```python
from build123d import *

# Parameters (mm, degrees)
BOSS_EXTRUDE1_DEPTH = 2.5
CUT_EXTRUDE1_REACH  = 26.645
SKETCH2_R           = 1.715
SKETCH2_R_2         = 8.98
SKETCH3_R           = 2.6543
BOSS_EXTRUDE2_DEPTH = 70.305
BOSS_EXTRUDE3_START = 4
SKETCH4_R           = 21
SKETCH4_R_2         = 8.98
BOSS_EXTRUDE3_DEPTH = 4
SKETCH6_R           = 21
SKETCH6_R_2         = 8.98
BOSS_EXTRUDE4_DEPTH = 2
CUT_EXTRUDE3_START  = -15
SKETCH7_R           = 1.715
CUT_EXTRUDE3_DEPTH  = 15
SKETCH8_R           = 8.98
CUT_EXTRUDE4_DEPTH  = 2
SKETCH9_R           = 11.0744
SKETCH9_R_2         = 8.98
BOSS_EXTRUDE5_DEPTH = 2.35


with BuildPart() as part:
    # Sketch1 → Boss-Extrude1 (new body)
    with BuildSketch(Plane(origin=(0, 0, 0), x_dir=(1, 0, 0), z_dir=(0, 1, 0))):
        with BuildLine():
            Line((0.597960958, 12.236443242), (0.597960958, 17.5133))
            Line((0.597960958, 17.5133), (-2.819411684, 17.5133))
            Line((-2.819411684, 17.5133), (-2.819411684, 11.976881697))
            ThreePointArc((-2.819411684, 11.976881697), (-9.752212861, 8.278991937), (-13.533031252, 1.391065316))
            ThreePointArc((-13.533031252, 1.391065316), (-17.156497956, -0.999626805), (-13.683409812, -3.603965207))
            ThreePointArc((-13.683409812, -3.603965207), (-10.042516815, -11.01106651), (-2.819411684, -15.004561697))
            Line((-2.819411684, -15.004561697), (-2.819411684, -17.5133))
            Line((-2.819411684, -17.5133), (0.597960958, -17.5133))
            Line((0.597960958, -17.5133), (0.597960958, -15.264123242))
            ThreePointArc((0.597960958, -15.264123242), (9.161591247, -11.721092084), (13.538839655, -3.55233882))
            ThreePointArc((13.538839655, -3.55233882), (17.156522938, -1.000460972), (13.393344487, 1.331534062))
            ThreePointArc((13.393344487, 1.331534062), (8.853545908, 8.96396608), (0.597960958, 12.236443242))
        make_face()
    extrude(amount=BOSS_EXTRUDE1_DEPTH)

    # Sketch2 → Cut-Extrude1 (cut, up to next)
    with BuildSketch(Plane(origin=(0, 2.5, 0), x_dir=(1, 0, 0), z_dir=(0, 1, 0)), mode=Mode.PRIVATE) as cut_extrude1_sk1:
        with Locations(Location((-14.5034, -1.0795, 0), (0, 0, 270))):
            Circle(SKETCH2_R)
    cut_extrude1_tool1 = extrude(cut_extrude1_sk1.sketch, amount=-CUT_EXTRUDE1_REACH, mode=Mode.PRIVATE) & part.part
    # Sketch2 → Cut-Extrude1 (cut, up to next)
    with BuildSketch(Plane(origin=(0, 2.5, 0), x_dir=(1, 0, 0), z_dir=(0, 1, 0)), mode=Mode.PRIVATE) as cut_extrude1_sk2:
        with Locations(Location((14.5034, -1.0795, 0), (0, 0, 270))):
            Circle(SKETCH2_R)
    cut_extrude1_tool2 = extrude(cut_extrude1_sk2.sketch, amount=-CUT_EXTRUDE1_REACH, mode=Mode.PRIVATE) & part.part
    # Sketch2 → Cut-Extrude1 (cut, up to next)
    with BuildSketch(Plane(origin=(0, 2.5, 0), x_dir=(1, 0, 0), z_dir=(0, 1, 0)), mode=Mode.PRIVATE) as cut_extrude1_sk3:
        with Locations(Location((-0.0762, -1.51384, 0), (0, 0, 270))):
            Circle(SKETCH2_R_2)
    cut_extrude1_tool3 = extrude(cut_extrude1_sk3.sketch, amount=-CUT_EXTRUDE1_REACH, mode=Mode.PRIVATE) & part.part
    add(cut_extrude1_tool1.solids().sort_by_distance((-14.5034, 2.5, 1.0795))[0], mode=Mode.SUBTRACT)
    add(cut_extrude1_tool2.solids().sort_by_distance((14.5034, 2.5, 1.0795))[0], mode=Mode.SUBTRACT)
    add(cut_extrude1_tool3.solids().sort_by_distance((-0.0762, 2.5, 1.51384))[0], mode=Mode.SUBTRACT)

    # Sketch3 → Boss-Extrude2 (add)
    with BuildSketch(Plane(origin=(0, 2.5, 0), x_dir=(1, 0, 0), z_dir=(0, 1, 0))):
        with Locations(Location((-14.5034, -1.0795, 0), (0, 0, 68.556492541))):
            Circle(SKETCH3_R)
        with Locations(Location((14.5034, -1.0795, 0), (0, 0, 114.72164566))):
            Circle(SKETCH3_R)
    extrude(amount=BOSS_EXTRUDE2_DEPTH)

    # Sketch4 → Boss-Extrude3 (add)
    with BuildSketch(Plane(origin=(0, 72.805, 0), x_dir=(1, 0, 0), z_dir=(0, 1, 0)).offset(BOSS_EXTRUDE3_START)):
        with Locations(Location((-0.0762, -1.51384, 0), (0, 0, 270))):
            Circle(SKETCH4_R)
        with Locations(Location((-0.0762, -1.51384, 0), (0, 0, 270))):
            Circle(SKETCH4_R_2, mode=Mode.SUBTRACT)
    extrude(amount=-BOSS_EXTRUDE3_DEPTH)

    # Sketch6 → Boss-Extrude4 (add)
    with BuildSketch(Plane(origin=(0, 37.805, 0), x_dir=(-1, 0, 0), z_dir=(0, -1, 0))):
        with Locations(Location((0.0762, -1.51384, 0), (0, 0, 90))):
            Circle(SKETCH6_R)
        with Locations(Location((0.0762, -1.51384, 0), (0, 0, 270))):
            Circle(SKETCH6_R_2, mode=Mode.SUBTRACT)
    extrude(amount=BOSS_EXTRUDE4_DEPTH)

    # Sketch7 → Cut-Extrude3 (cut)
    with BuildSketch(Plane.XZ.offset(CUT_EXTRUDE3_START)):
        with Locations(Location((-14.5034, 1.0795, 0), (0, 0, 90))):
            Circle(SKETCH7_R)
        with Locations(Location((14.5034, 1.0795, 0), (0, 0, 90))):
            Circle(SKETCH7_R)
    extrude(amount=CUT_EXTRUDE3_DEPTH, mode=Mode.SUBTRACT)

    # Sketch8 → Cut-Extrude4 (cut)
    with BuildSketch(Plane(origin=(0, 76.805, 0), x_dir=(1, 0, 0), z_dir=(0, 1, 0))):
        with BuildLine():
            Line((-10.0762, -1.51384), (-7.3262, -15.51384))
            ThreePointArc((-7.3262, -15.51384), (-0.0762, -17.51384), (7.1738, -15.51384))
            Line((7.1738, -15.51384), (9.9238, -1.51384))
            Line((9.9238, -1.51384), (7.1738, 12.48616))
            ThreePointArc((7.1738, 12.48616), (-0.0762, 14.48616), (-7.3262, 12.48616))
            Line((-7.3262, 12.48616), (-10.0762, -1.51384))
        make_face()
        with Locations(Location((-0.0762, -1.51384, 0), (0, 0, 270))):
            Circle(SKETCH8_R, mode=Mode.SUBTRACT)
    extrude(amount=-CUT_EXTRUDE4_DEPTH, mode=Mode.SUBTRACT)

    # Sketch9 → Boss-Extrude5 (add)
    with BuildSketch(Plane.XZ):
        with Locations(Location((-0.0762, 1.51384, 0), (0, 0, 90))):
            Circle(SKETCH9_R)
        with Locations(Location((-0.0762, 1.51384, 0), (0, 0, 90))):
            Circle(SKETCH9_R_2, mode=Mode.SUBTRACT)
    extrude(amount=BOSS_EXTRUDE5_DEPTH)


solid = part.part
```
Here's how the part is built. I have some questions about the finished solid (model axes, mm). A direction names the side the tool comes from. Coordinates: 2 decimals unless noted, no trailing zeros. Loops run counter-clockwise (first coordinate to the right, second up) from the corner with the lowest first, then second, coordinate; pieces in that order, holes last. Notation, with made-up numbers: (24.25, 59) -> (71.25, 59) arc R11 cw to (71.25, 79) -> close; hole circle Ø10 at (-29.5, 83). An arc over 180 degrees is marked (long way). Return JSON: item names as keys, results as strings.
1) For faces 5 (the face through (-1, 1, -17.513)), 6 (the face through (-7, 74.805, 8)), 7 (the face through (0.598, 1, -15)), 8 (the face through (-1, 1, 17.513)), 9 (the face through (-17.08, 55.06, 0.44)), which set-ups out of +Z, -Z, +X, -X, +Y, -Y let a thin tool reach every point of the face, with its end or its side?
Results below:
{"face 5": "-Z, +X, -X, -Y", "face 6": "+Y", "face 7": "-Z, +X, -Y", "face 8": "+Z, +X, -X, -Y", "face 9": "none"}
2) If we section it at D-D, the plane y = 11.5: Write out the boundary of the cut face in (x, z) (1 decimal).
Results below:
{"outline": "circle Ø5.3 at (-14.5, 1.1); circle Ø5.3 at (14.5, 1.1); hole circle Ø3.4 at (-14.5, 1.1); hole circle Ø3.4 at (14.5, 1.1)"}
3) If we section it at B-B, the plane x = -6: Count the separate pieces of the cut face and the enclosed holes in it, then the cut area to 3 significant figures.
Results below:
{"separate pieces": "6", "enclosed holes": "0", "area": "170 mm²"}
4) Will these pins go through, and if not, where does the flat tip stop? pin 1 (2.5 mm diameter, centred on x = -14, z = 1.5, fed in from -Y); pin 2 (2 mm diameter, centred on y = 68.5, z = 3, fed in from +X); pin 3 (12 mm diameter, centred on y = 22, z = 4, fed in from +X); pin 4 (5 mm diameter, centred on x = -3, z = -14, fed in from +Y) (3 decimals).
Results below:
{"pin 1": "y = 0", "pin 2": "x = 16.99", "pin 3": "x = 17.16", "pin 4": "y = 76.805"}
5) Thinking about a two-plate mould opening in Y: for faces 1 (the face through (10, 76.805, 6)), 2 (the face through (9, 2.5, 0)), 3 (the face through (20.745, 36.819, 4.248)), 4 (the face through (-15, 15, 1)), which applies, +Y half, -Y half, draft (parallel to the pull), parting line (faces both ways), or undercut?
Results below:
{"face 1": "+Y half", "face 2": "undercut", "face 3": "draft", "face 4": "-Y half"}
6) I need wall thicknesses on line 1 (Y direction, x = 9, z = 9) (3 decimals); line 2 (Y direction, x = -4, z = -9.5) (3 decimals); line 3 (Y direction, x = -15, z = -13) (3 decimals). Which ranges of each line are inside material? Lowest first, please. Write a range as from..to.
Results below:
{"line 1": "0..2.5, 35.805..37.805, 72.805..76.805", "line 2": "0..2.5, 35.805..37.805, 72.805..74.805", "line 3": "35.805..37.805, 72.805..76.805"}
7) If we section it at A-A, the plane z = -11: Write out the boundary of the cut face in (x, y) (3 decimals).
Results below:
{"outline": "(-16.94, 35.805) -> (16.788, 35.805) -> (16.788, 37.805) -> (-16.94, 37.805) -> close; (-16.94, 72.805) -> (16.788, 72.805) -> (16.788, 76.805) -> (7.466, 76.805) -> (7.466, 74.805) -> (-7.618, 74.805) -> (-7.618, 76.805) -> (-16.94, 76.805) -> close; (-5.815, 0) -> (5.662, 0) -> (5.662, 2.5) -> (-5.815, 2.5) -> close"}
